Model file for the job. Use its own axes, mm. Face numbers are marked on the shaded views. A direction names the side the tool comes from. Round coordinates to 2 decimals unless told otherwise and drop trailing zeros. Order: outer loops, then holes, each group sorted by start corner. A loop starts at its lowest first (then second) coordinate and runs counter-clockwise, first axis right, second up. Notation, with made-up numbers: M 11,57 L 51,57 A19 cw 51,94 Z; hole C 52,-28.5 d11. An arc over 180 degrees is marked long. Return JSON: item names as keys, results as strings. Group by question number.
Item 1: Slice it at A-A on z = -13. Give the number of separate pieces and of enclosed holes in the cut face, then the cut area to 3 significant figures.
Item 2: Slice it at C-C on x = -9. Write the cut outline in (y, z).
Item 3: Which spindle directions (+Z, -Z, +X, -X, +Y, -Y) get a long thin tool onto all of the face, cutting with end or side? Do the marked faces 1, 2, 3, 4 and 5. Say none if no direction does.
Item 4: Probe line 1 along Z through (x, y) = (-32, -3); line 2 along Z through (x, y) = (-32.5, -25); line 3 along Y through (x, z) = (-1, 8.5). List the from-to ranges inside material, lowest first.
Item 5: Slice it at B-B on y = 0. Write the cut outline in (x, z), then the cut area to 3 significant figures.
Item 6: Pull direction Z, two halves, no side cores. Call the marked faces 6, 7 and 8: pulls with the +Z half, pulls with the -Z half, needs draft (parallel to the pull), parting line crosses it, or undercut.
Item 7: Slice it at D-D on z = 5. Write the cut outline in (x, y) (1 decimal), then the cut area to 3 significant figures.
Item 8: Pin check, flat tips, straight feed: pin 1 Ø1 at (y, z) = (-2.5, 15) entering from +X; pin 2 Ø4 at (y, z) = (-11, 10) entering from +X; pin 3 Ø3 at (x, y) = (22, -31) entering from +Z; pin 4 Ø5 at (x, z) = (-42.5, 14.5) entering from -Y. Stop position of each tip, or through.
from build123d import *

# Parameters (mm, degrees)
ESQUISSE1_R             = 1.6
BOSS_EXTRU_1_DEPTH      = 10
ESQUISSE2_R             = 32.8
BOSS_EXTRU_2_DEPTH      = 22
ENL_V_MAT_EXTRU_1_DEPTH = 3.5
BOSS_EXTRU_3_REACH      = 12
ESQUISSE4_R             = 32.8
ESQUISSE5_R             = 16
BOSS_EXTRU_4_DEPTH      = 19
ESQUISSE6_R             = 1
BOSS_EXTRU_5_DEPTH      = 27
BOSS_EXTRU_6_DEPTH      = 1.5
ESQUISSE8_R             = 5
BOSS_EXTRU_7_DEPTH      = 5.5


with BuildPart() as part:
    # Esquisse1 → Boss.-Extru.1 (new body)
    with BuildSketch(Plane.XY):
        with BuildLine():
            ThreePointArc((-56.3, -16.861494596), (-60.528670487, -14.599558136), (-64.01, -11.301322931))
            ThreePointArc((-64.01, -11.301322931), (-65, 0), (-64.01, 11.301322931))
            ThreePointArc((-64.01, 11.301322931), (-60.528670487, 14.599558136), (-56.3, 16.861494596))
            Line((-56.3, 16.861494596), (-39.624688626, 23.091930519))
            ThreePointArc((-39.624688626, 23.091930519), (-36.690940127, 29.525679018), (-30.257191628, 26.591930519))
            Line((-30.257191628, 26.591930519), (-12.425, 33.254614341))
            ThreePointArc((-12.425, 33.254614341), (1.381675102, 35.473102119), (14.973963383, 32.187426436))
            Line((14.973963383, 32.187426436), (20.756023105, 34.801647207))
            ThreePointArc((20.756023105, 34.801647207), (24.347774736, 34.238511045), (26, 31))
            Line((26, 31), (25.359978077, 24.841930519))
            ThreePointArc((25.359978077, 24.841930519), (35.5, 0), (25.359978077, -24.841930519))
            Line((25.359978077, -24.841930519), (26, -31))
            ThreePointArc((26, -31), (24.347774736, -34.238511045), (20.756023105, -34.801647207))
            Line((20.756023105, -34.801647207), (14.973963383, -32.187426436))
            ThreePointArc((14.973963383, -32.187426436), (1.381675102, -35.473102119), (-12.425, -33.254614341))
            Line((-12.425, -33.254614341), (-30.257191628, -26.591930519))
            ThreePointArc((-30.257191628, -26.591930519), (-36.690940127, -29.525679018), (-39.624688626, -23.091930519))
            Line((-39.624688626, -23.091930519), (-56.3, -16.861494596))
        make_face()
        with Locations((-35, -25)):
            Circle(ESQUISSE1_R, mode=Mode.SUBTRACT)
        with Locations((22, 31)):
            Circle(ESQUISSE1_R, mode=Mode.SUBTRACT)
        with Locations((-35, 25)):
            Circle(ESQUISSE1_R, mode=Mode.SUBTRACT)
        with Locations((22, -31)):
            Circle(ESQUISSE1_R, mode=Mode.SUBTRACT)
    extrude(amount=BOSS_EXTRU_1_DEPTH)

    # Esquisse2 → Boss.-Extru.2 (add)
    with BuildSketch(Plane.XY.offset(10)):
        Circle(ESQUISSE2_R)
    extrude(amount=BOSS_EXTRU_2_DEPTH)

    # Esquisse3 → Enlèv. mat.-Extru.1 (cut)
    with BuildSketch(Plane.XY.offset(10)):
        with BuildLine():
            Line((-55.775, -15.456370046), (-37.378202776, -22.330008789))
            ThreePointArc((-37.378202776, -22.330008789), (-36.165940127, -28.120554469), (-31.453677478, -24.543603151))
            Line((-31.453677478, -24.543603151), (-11.9, -31.849489792))
            ThreePointArc((-11.9, -31.849489792), (1.664031028, -33.959255009), (14.956816294, -30.533484019))
            Line((14.956816294, -30.533484019), (21.291141631, -33.397398551))
            ThreePointArc((21.291141631, -33.397398551), (23.468656713, -33.023128137), (24.499056843, -31.06866508))
            Line((24.499056843, -31.06866508), (23.79417774, -24.286562245))
            ThreePointArc((23.79417774, -24.286562245), (34, 0), (23.79417774, 24.286562245))
            Line((23.79417774, 24.286562245), (24.499056843, 31.06866508))
            ThreePointArc((24.499056843, 31.06866508), (23.468656713, 33.023128137), (21.291141631, 33.397398551))
            Line((21.291141631, 33.397398551), (14.956816294, 30.533484019))
            ThreePointArc((14.956816294, 30.533484019), (1.664031028, 33.959255009), (-11.9, 31.849489792))
            Line((-11.9, 31.849489792), (-31.453677478, 24.543603151))
            ThreePointArc((-31.453677478, 24.543603151), (-36.165940127, 28.120554469), (-37.378202776, 22.330008789))
            Line((-37.378202776, 22.330008789), (-55.775, 15.456370046))
            ThreePointArc((-55.775, 15.456370046), (-59.496201473, 13.493411636), (-62.6, 10.653168543))
            ThreePointArc((-62.6, 10.653168543), (-63.5, 0), (-62.6, -10.653168543))
            ThreePointArc((-62.6, -10.653168543), (-59.496201473, -13.493411636), (-55.775, -15.456370046))
        make_face()
    extrude(amount=-ENL_V_MAT_EXTRU_1_DEPTH, mode=Mode.SUBTRACT)

    # Esquisse4 → Boss.-Extru.3 (add, up to next)
    with BuildSketch(Plane(origin=(0, 0, 10), x_dir=(-1, 0, 0), z_dir=(0, 0, -1)), mode=Mode.PRIVATE) as boss_extru_3_sk1:
        Circle(ESQUISSE4_R)
    boss_extru_3_tool1 = extrude(boss_extru_3_sk1.sketch, amount=BOSS_EXTRU_3_REACH, mode=Mode.PRIVATE) - part.part
    add(boss_extru_3_tool1.solids().sort_by_distance((0, 0, 10))[0])

    # Esquisse5 → Boss.-Extru.4 (add)
    with BuildSketch(Plane(origin=(0, 0, 0), x_dir=(-1, 0, 0), z_dir=(0, 0, -1))):
        with Locations((50, 0)):
            Circle(ESQUISSE5_R)
    extrude(amount=BOSS_EXTRU_4_DEPTH)

    # Esquisse6 → Boss.-Extru.5 (add)
    with BuildSketch(Plane(origin=(0, 0, 0), x_dir=(-1, 0, 0), z_dir=(0, 0, -1))):
        Polygon((-20.489225606, -29.008126327), (-22.969626005, -28.695694159), (-24.480400399, -30.687567832), (-23.510774394, -32.991873673), (-21.030373995, -33.304305841), (-19.519599601, -31.312432168), align=None)
        with Locations((-22, -31)):
            Circle(ESQUISSE6_R, mode=Mode.SUBTRACT)
        Polygon((36.086835018, -22.748602735), (33.593650283, -22.933074633), (32.506815266, -25.184471898), (33.913164982, -27.251397265), (36.406349717, -27.066925367), (37.493184734, -24.815528102), align=None)
        with Locations((35, -25)):
            Circle(ESQUISSE6_R, mode=Mode.SUBTRACT)
        Polygon((36.720274889, 26.814016072), (34.289153443, 27.396809791), (32.568878555, 25.582793719), (33.279725111, 23.185983928), (35.710846557, 22.603190209), (37.431121445, 24.417206281), align=None)
        with Locations((35, 25)):
            Circle(ESQUISSE6_R, mode=Mode.SUBTRACT)
        Polygon((-19.952160425, 32.43399898), (-22.217959758, 33.490480585), (-24.265799333, 32.056481605), (-24.047839575, 29.56600102), (-21.782040242, 28.509519415), (-19.734200667, 29.943518395), align=None)
        with Locations((-22, 31)):
            Circle(ESQUISSE6_R, mode=Mode.SUBTRACT)
    extrude(amount=BOSS_EXTRU_5_DEPTH)

    # Esquisse7 → Boss.-Extru.6 (add)
    with BuildSketch(Plane(origin=(0, 0, -8), x_dir=(-1, 0, 0), z_dir=(0, 0, -1))):
        with BuildLine():
            Line((30.257191628, 26.591930519), (12.425, 33.254614341))
            ThreePointArc((12.425, 33.254614341), (-1.381675102, 35.473102119), (-14.973963383, 32.187426436))
            Line((-14.973963383, 32.187426436), (-20.756023105, 34.801647207))
            ThreePointArc((-20.756023105, 34.801647207), (-24.347774736, 34.238511045), (-26, 31))
            Line((-26, 31), (-25.359978077, 24.841930519))
            ThreePointArc((-25.359978077, 24.841930519), (-35.5, 0), (-25.359978077, -24.841930519))
            Line((-25.359978077, -24.841930519), (-26, -31))
            ThreePointArc((-26, -31), (-24.347774736, -34.238511045), (-20.756023105, -34.801647207))
            Line((-20.756023105, -34.801647207), (-14.973963383, -32.187426436))
            ThreePointArc((-14.973963383, -32.187426436), (-1.381675102, -35.473102119), (12.425, -33.254614341))
            Line((12.425, -33.254614341), (30.257191628, -26.591930519))
            ThreePointArc((30.257191628, -26.591930519), (36.690940127, -29.525679018), (39.624688626, -23.091930519))
            ThreePointArc((39.624688626, -23.091930519), (33.487603548, 0), (39.624688626, 23.091930519))
            ThreePointArc((39.624688626, 23.091930519), (36.690940127, 29.525679018), (30.257191628, 26.591930519))
        make_face()
    extrude(amount=BOSS_EXTRU_6_DEPTH)

    # Esquisse8 → Boss.-Extru.7 (add)
    with BuildSketch(Plane.XY.offset(6.5)):
        with Locations((-50, 0)):
            Circle(ESQUISSE8_R)
    extrude(amount=BOSS_EXTRU_7_DEPTH)


solid = part.part
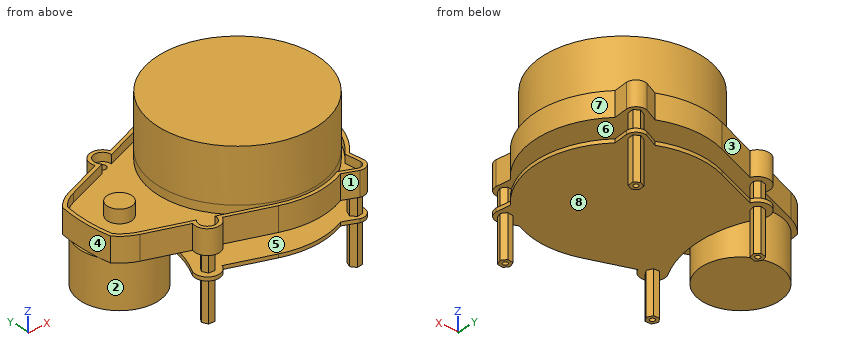
Output values:
{
 "1": {"separate pieces": "5", "enclosed holes": "4", "area": "857 mm²"},
 "2": {"outline": "M -34.34,-9.5 L 34.34,-9.5 L 34.34,-8 L -34.34,-8 Z; M -34.34,0 L 34.34,0 L 34.34,10 L 32.79,10 L 32.79,6.5 L 31.54,6.5 L 31.54,32 L -31.54,32 L -31.54,6.5 L -32.79,6.5 L -32.79,10 L -34.34,10 Z"},
 "3": {"face 1": "+Z, -Z, -Y", "face 2": "-Z", "face 3": "+Z, -Z, +Y", "face 4": "+Z, -X", "face 5": "none"},
 "4": {"line 1": "-9.5 to -8, 0 to 32", "line 2": "-9.5 to -8, 0 to 6.5", "line 3": "-35.49 to -33.99, -32.78 to 32.78, 33.99 to 35.49"},
 "5": {"outline": "M -66,-19 L -34,-19 L -34,0 L 35.5,0 L 35.5,10 L 34,10 L 34,6.5 L 32.8,6.5 L 32.8,32 L -32.8,32 L -32.8,6.5 L -45,6.5 L -45,12 L -55,12 L -55,6.5 L -63.5,6.5 L -63.5,10 L -65,10 L -65,0 L -66,0 Z; M -33.49,-9.5 L 35.5,-9.5 L 35.5,-8 L -33.49,-8 Z", "area": "3,100 mm²"},
 "6": {"face 6": "undercut", "face 7": "needs draft", "face 8": "pulls with the -Z half"},
 "7": {"outline": "M -64,-11.3 A18 ccw -56.3,-16.9 L -39.6,-23.1 A5 ccw -30.3,-26.6 L -12.4,-33.3 A35.5 ccw 15,-32.2 L 20.8,-34.8 A4 ccw 26,-31 L 25.4,-24.8 A35.5 ccw 25.4,24.8 L 26,31 A4 ccw 20.8,34.8 L 15,32.2 A35.5 ccw -12.4,33.3 L -30.3,26.6 A5 ccw -39.6,23.1 L -56.3,16.9 A18 ccw -64,11.3 A65 ccw Z; hole C -35,-25 d3.2; hole C -35,25 d3.2; hole C 22,-31 d3.2; hole C 22,31 d3.2", "area": "5,440 mm²"},
 "8": {"pin 1": "x = 32.74", "pin 2": "x = 34.34", "pin 3": "z = 0", "pin 4": "through"}
}
